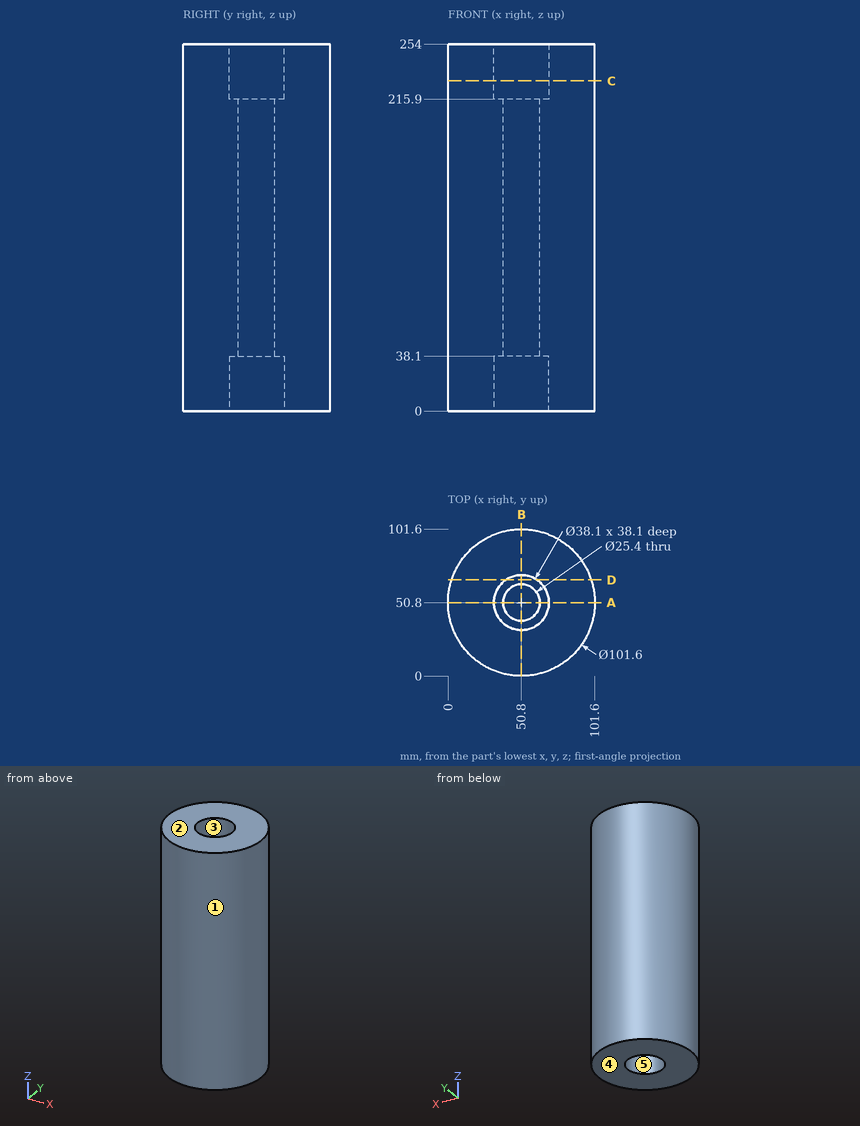
Could you check a few things on this drawing? It's one solid part, dimensions in mm from its lowest x, y, z. A direction names the side the tool comes from. Round coordinates to 2 decimals unless told otherwise and drop trailing zeros. Order: outer loops, then holes, each group sorted by start corner. A loop starts at its lowest first (then second) coordinate and runs counter-clockwise, first axis right, second up. Notation, with made-up numbers: M 2.25,-24.75 L 35.25,-24.75 A4 cw 35.25,-18.75 Z; hole C -19.75,62 d8. An arc over 180 degrees is marked long. Return JSON: item names as keys, results as strings. Group by question number.
1. On a 3-axis mill with a long thin cutter (end or side, diameter ignored), from which of +Z, -Z, +X, -X, +Y, -Y can I reach the whole of each face in a straight line? I mean the marked faces 4 and 5. Say none if no direction works.
2. If we section it at A-A on y = 50.8: List the corners of the cut face in (x, z) for me, then the cut area to 3 significant figures.
3. If we section it at C-C on z = 228.5: List the corners of the cut face in (x, y) for me, then the cut area to 3 significant figures.
4. If we section it at D-D on y = 66.5: List the corners of the cut face in (x, z) for me.
5. If we mould it in two halves opening along Y, with no side actions, what happens to the marked faces 1, 2 and 3? For each: pulls with the +Y half, pulls with the -Y half, needs draft (parallel to the pull), parting line crosses it, or undercut.
6. I'm going to push flat-ended pins straight in: pin 1 Ø11.5 at (x, y) = (45, 46) entering from +Z; pin 2 Ø23 at (x, y) = (50.8, 50.8) entering from -Z; pin 3 Ø1 at (x, z) = (53.5, 148) entering from +Y; pin 4 Ø5 at (x, z) = (80.5, 218.5) entering from -Y. Where does each tip first touch, or does it pass through?
7. Please list where these lines run through material, in increasing order: probe 1 along Y at (x, z) = (50, 16); probe 2 along X at (y, z) = (50.8, 9); probe 3 along X at (y, z) = (50, 126).
Reply:
{
 "1": {"face 4": "-Z, +X, -X, +Y, -Y", "face 5": "-Z"},
 "2": {"outline": "M 0,0 L 31.75,0 L 31.75,38.1 L 38.1,38.1 L 38.1,215.9 L 31.75,215.9 L 31.75,254 L 0,254 Z; M 63.5,38.1 L 69.85,38.1 L 69.85,0 L 101.6,0 L 101.6,254 L 69.85,254 L 69.85,215.9 L 63.5,215.9 Z", "area": "18,400 mm^2"},
 "3": {"outline": "C 50.8,50.8 d101.6; hole C 50.8,50.8 d38.1", "area": "6,970 mm^2"},
 "4": {"outline": "M 2.49,0 L 40.01,0 L 40.01,38.1 L 61.59,38.1 L 61.59,0 L 99.11,0 L 99.11,254 L 61.59,254 L 61.59,215.9 L 40.01,215.9 L 40.01,254 L 2.49,254 Z"},
 "5": {"face 1": "parting line crosses it", "face 2": "needs draft", "face 3": "undercut"},
 "6": {"pin 1": "z = 215.9", "pin 2": "through", "pin 3": "y = 101.55", "pin 4": "y = 7.9"},
 "7": {"probe 1": "0.01 to 31.77, 69.83 to 101.59", "probe 2": "0 to 31.75, 69.85 to 101.6", "probe 3": "0.01 to 38.13, 63.47 to 101.59"}
}
